Read the model definition and answer for the solid it produces. Units are mm, in the model's axes. Face numbers are marked on the shaded views. Coordinates: 2 decimals unless noted, no trailing zeros. Write each loop counter-clockwise with the first axis right and the second up, starting at its lowest first coordinate (ties: lowest second). Pieces come first, ordered by that corner, then holes.
Item 1: Section D-D (x = 4) is taken. Give the vertices of the cut face in (y, z).
Item 2: Determine the mould class of the marked faces 1 and 2 for opening direction Y: released by +Y, released by -Y, zero draft, split by the parting line, or undercut.
Item 3: Section B-B (z = -3.75) is taken. Give the vertices of the cut face in (x, y).
Item 4: Each of these flat-tipped pins is pushed along its axis until it touches: P1, Ø1, axis at x = 110, z = -4, coming from the -Y side; P2, Ø5, axis at y = -74, z = -6.5, coming from the +X side; P3, Ø1, axis at y = -21, z = -3.5, coming from the -X side; P4, Ø10, axis at x = 60, y = -58.5, coming from the -Z side. Where does it stop, or does it pass through?
Item 5: Section C-C (y = -119) is taken. Give the vertices of the cut face in (x, z), then the cut area to 3 significant figures.
Item 6: Straight lines are drawn through the part: probe 1 along X at (y, z) = (-104, -6.25); probe 2 along Y at (x, z) = (-4, -4.75); probe 3 along Z at (x, y) = (-8.5, -42.5). For each, find the intervals that lie inside material, in ascending order.
Item 7: Section A-A (x = 61) is taken. Give the vertices of the cut face in (y, z), then the cut area to 3 significant figures.
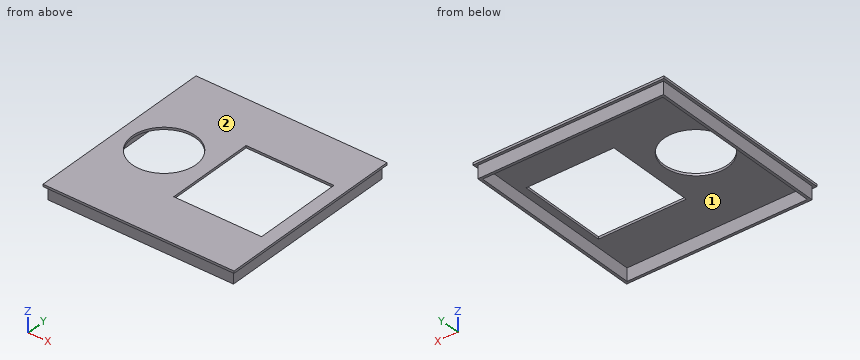
from build123d import *

# Parameters (mm, degrees)
CROQUIS1_W              = 150
CROQUIS1_H              = 150
CROQUIS1_R              = 25
CROQUIS1_W_2            = 69
CROQUIS1_H_2            = 71
SALIENTE_EXTRUIR1_DEPTH = 1.8
CROQUIS2_W              = 145.8
CROQUIS2_H              = 145.8
CROQUIS2_W_2            = 141.6
CROQUIS2_H_2            = 141.6
SALIENTE_EXTRUIR2_DEPTH = 10


with BuildPart() as part:
    # Croquis1 → Saliente-Extruir1 (new body)
    with BuildSketch(Plane.XY):
        with Locations((57.57534771, -67.552941176)):
            Rectangle(CROQUIS1_W, CROQUIS1_H)
        with Locations((17.57534771, -67.552941176)):
            Circle(CROQUIS1_R, mode=Mode.SUBTRACT)
        with Locations((88.07534771, -67.552941176)):
            Rectangle(CROQUIS1_W_2, CROQUIS1_H_2, mode=Mode.SUBTRACT)
    extrude(amount=SALIENTE_EXTRUIR1_DEPTH)

    # Croquis2 → Saliente-Extruir2 (add)
    with BuildSketch(Plane(origin=(0, 0, 0), x_dir=(-1, 0, 0), z_dir=(0, 0, -1))):
        with Locations((-57.57534771, -67.552941176)):
            Rectangle(CROQUIS2_W, CROQUIS2_H)
        with Locations((-57.57534771, -67.552941176)):
            Rectangle(CROQUIS2_W_2, CROQUIS2_H_2, mode=Mode.SUBTRACT)
    extrude(amount=SALIENTE_EXTRUIR2_DEPTH)


solid = part.part
Established:
1. outline: (-142.55, 0) - (-140.45, 0) - (-140.45, -10) - (-138.35, -10) - (-138.35, 0) - (-88.55, 0) - (-88.55, 1.8) - (-142.55, 1.8) - close; (-46.56, 0) - (3.25, 0) - (3.25, -10) - (5.35, -10) - (5.35, 0) - (7.45, 0) - (7.45, 1.8) - (-46.56, 1.8) - close
2. face 1: undercut
2. face 2: zero draft
3. outline: (-15.32, -140.45) - (130.48, -140.45) - (130.48, 5.35) - (-15.32, 5.35) - close; hole (-13.22, -138.35) - (128.38, -138.35) - (128.38, 3.25) - (-13.22, 3.25) - close
4. P1: stops at y = -140.45
4. P2: stops at x = 130.48
4. P3: stops at x = -15.32
4. P4: passes through
5. outline: (-17.42, 0) - (-15.32, 0) - (-15.32, -10) - (-13.22, -10) - (-13.22, 0) - (128.38, 0) - (128.38, -10) - (130.48, -10) - (130.48, 0) - (132.58, 0) - (132.58, 1.8) - (-17.42, 1.8) - close
5. area: 312 mm2
6. probe 1: x = -15.32 to -13.22, 128.38 to 130.48
6. probe 2: y = -140.45 to -138.35, 3.25 to 5.35
6. probe 3: z = 0 to 1.8
7. outline: (-142.55, 0) - (-140.45, 0) - (-140.45, -10) - (-138.35, -10) - (-138.35, 0) - (-103.05, 0) - (-103.05, 1.8) - (-142.55, 1.8) - close; (-32.05, 0) - (3.25, 0) - (3.25, -10) - (5.35, -10) - (5.35, 0) - (7.45, 0) - (7.45, 1.8) - (-32.05, 1.8) - close
7. area: 184 mm2
